Work out the finished part from the listing and answer in its coordinate system (mm). Give positions to 0.01 mm unless a question says otherwise; leave off trailing zeros. Loops run counter-clockwise (first coordinate to the right, second up) from the corner with the lowest first, then second, coordinate; pieces in that order, holes last. Notation, with made-up numbers: M 51.5,-27 L 59.5,-27 A21 ccw 59.5,4 Z; hole C 88.5,48 d4. An arc over 180 degrees is marked long. Answer as a JSON object with one key per item and string values. Group by question number.
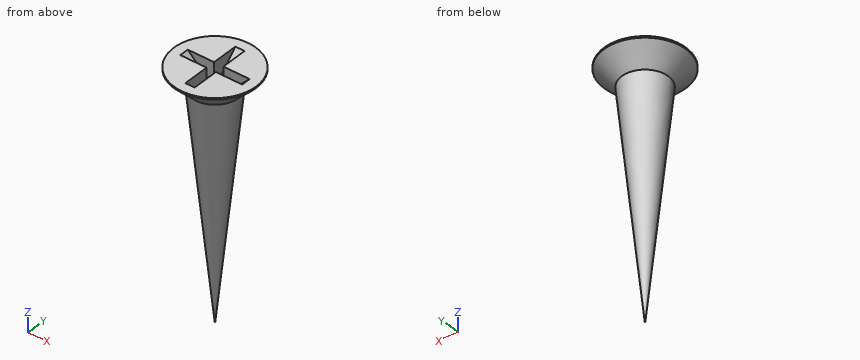
```python
from build123d import *

# Parameters (mm, degrees)
POCKET017_DEPTH    = 0.3
POLARPATTERN_COUNT = 2
POLARPATTERN_ANGLE = 90


with BuildPart() as part:
    # Sketch057 → Revolution010 (revolve)
    with BuildSketch(Plane.XZ):
        Polygon((0, 0), (0, -16), (1.5, -1.25), (2.65, -0.1), (2.65, 0), align=None)
    revolve(axis=Axis((0, 0, 0), (0, 0, 1)))

    # Sketch058 → Pocket017 (cut, symmetric)
    with BuildSketch(Plane.XZ):
        Polygon((-2, 0), (0, -2), (2, 0), align=None)
    pocket017 = extrude(amount=POCKET017_DEPTH, both=True, mode=Mode.SUBTRACT)

    # PolarPattern: Pocket017 ×2 about axis
    polarpattern_axis = Axis((0, 0, 0), (0, 0, 1))
    for i in range(1, POLARPATTERN_COUNT):
        add(pocket017.rotate(polarpattern_axis, i * POLARPATTERN_ANGLE / (POLARPATTERN_COUNT - 1)), mode=Mode.SUBTRACT)


solid = part.part
```
Item 1: A cutting plane is placed at C-C (z = -4.75). Determine the outline of the cut face in (x, y).
Item 2: A cutting plane is placed at B-B (z = -11.75). Determine the outline of the cut face in (x, y), and give its area (3 significant figures).
Item 3: Find the intervals of material crossed by probe 1 along Y at (x, z) = (-0.95, -1); probe 2 along X at (y, z) = (-0.5, -9.5); probe 3 along X at (y, z) = (-2, -0.5), in increasing order. Write a range as [from, to].
Item 4: Given pin 1 Ø1.9 at (y, z) = (-1.5, -0.5) entering from +X; pin 2 Ø1.9 at (x, z) = (1, -0.5) entering from -Y; pin 3 Ø0.5 at (y, z) = (1, -1) entering from -X, each flat-ended and moving along its own axis, determine where each tip first touches the part or whether it passes through.
Item 5: A cutting plane is placed at A-A (z = -0.75). Determine the outline of the cut face in (x, y), and give its area (3 significant figures).
The answers:
{
 "1": {"outline": "C 0,0 d2.29"},
 "2": {"outline": "C 0,0 d0.86", "area": "0.587 mm^2"},
 "3": {"probe 1": "y = [-1.47, -0.3], [0.3, 1.47]", "probe 2": "x = [-0.43, 0.43]", "probe 3": "x = [-1.03, 1.03]"},
 "4": {"pin 1": "stops at x = 2.57", "pin 2": "stops at y = -2.65", "pin 3": "stops at x = -1.76"},
 "5": {"outline": "C 0,0 d4; hole M -1.25,-0.3 L -0.3,-0.3 L -0.3,-1.25 L 0.3,-1.25 L 0.3,-0.3 L 1.25,-0.3 L 1.25,0.3 L 0.3,0.3 L 0.3,1.25 L -0.3,1.25 L -0.3,0.3 L -1.25,0.3 Z", "area": "9.93 mm^2"}
}
